Autodesk Inventor part; units mm, degrees
ref_plane "YZ Plane" through (0, 0, 0) normal (1, 0, 0) x (0, 1, 0)
ref_plane "XZ Plane" through (0, 0, 0) normal (0, 1, 0) x (-1, 0, 0)
ref_plane "XY Plane" through (0, 0, 0) normal (0, 0, 1) x (1, 0, 0)
sketch "Sketch1" plane through (0, 0, 0) normal (0, 0, 1) x (1, 0, 0)
  line L0 (0, 0) -> (2.5, 0)
  line L1 (2.5, 0) -> (2.5, 8)
  line L2 (2.5, 8) -> (0, 8)
  line L3 (0, 8) -> (0, 0)
  line L4 (2.5, 8) -> (42, 8)
  line L5 (42, 8) -> (42, 0)
  line L6 (42, 0) -> (2.5, 0)
  line L7 (2.5, 0) -> (2.5, 8)
  circle A0 centre (42, 4) radius 2.5
  point P0 (42, 1.5)
  point P1 (42, 6.5)
  dimension "d0" = 8
  dimension "d1" = 2.5
  dimension "d2" = 39.5
  dimension "d3" = 5
revolve "Revolution1" add sketch "Sketch1" angle 360 about axis through (0, 8, 0) along (0, -1, 0) contours L1 L4 L5 A0 L6
sketch "Sketch2" plane through (0, 8, 0) normal (0, 1, 0) x (1, 0, 0)
  circle A0 centre (0, 0) radius 2.5
  circle A1 centre (0, 0) radius 30
  circle A2 centre (0, 0) radius 5
  line L0 (-4.3623, -2.4434) -> (-29.9003, -2.4434)
  line L1 (-4.3623, 2.4434) -> (-29.9003, 2.4434)
  line L2 (4.3623, 2.4434) -> (29.9003, 2.4434)
  line L3 (4.3623, -2.4434) -> (29.9003, -2.4434)
  line L4 (2.0546, -4.5583) -> (2.0546, -29.9296)
  line L5 (-2.0546, -4.5583) -> (-2.0546, -29.9296)
  line L6 (-2.0546, 4.5583) -> (-2.0546, 60.5512)
  line L7 (2.0546, 4.5583) -> (2.0546, 29.9296)
  point P0 (-2.0546, 29.9296)
  dimension "d5" = 60
  dimension "d6" = 10
extrude "Extrusion1" cut sketch "Sketch2" against normal blind 25 contours L2 A2 L7 A1 | A1 L4 A2 L3 | L6 A2 L1 A1 | A1 L0 A2 L5
properties part number "Roue_pami_V3"
Work out the finished part from the listing and answer in its coordinate system (mm). A direction names the side the tool comes from. Round coordinates to 2 decimals unless told otherwise and drop trailing zeros. Loops run counter-clockwise (first coordinate to the right, second up) from the corner with the lowest first, then second, coordinate; pieces in that order, holes last.
(1) The part is cut by section A-A, the plane x = 0. Give the vertices of the cut face in (y, z), and give its area (3 significant figures).
Computed values:
outline: (0, -42) - (1.5, -42) arc R2.5 cw to (6.5, -42) - (8, -42) - (8, -2.5) - (0, -2.5) - close; (0, 2.5) - (8, 2.5) - (8, 42) - (6.5, 42) arc R2.5 cw to (1.5, 42) - (0, 42) - close
area: 612 mm2
(2) The mould has two halves that part along Z. Classify faces 3 (the cylindrical face through (40.06, 7.24, 12.62)), 4 (the cylindrical face through (-3, 4, 4)), 5 (the flat face through (9, 8, 1)): pulls with the +Z half, pulls with the -Z half, needs draft (parallel to the pull), parting line crosses it, or undercut.
Computed values:
face 3: parting line crosses it
face 4: undercut
face 5: needs draft
(3) For faces 1 (the cylindrical face through (-20.86, 4.06, -21.56)), 2 (the flat face through (9, 0, 1)), determine the directions among +Z, -Z, +X, -X, +Y, -Y from which every point of the face is accessible in a straight line to the end or side of a thin tool.
Computed values:
face 1: +Y, -Y
face 2: +Z, -Z, +X, -X, -Y
(4) Find the intervals of material crossed by L1, parallel to Z at x = 5, y = 7.5; L2, parallel to X at y = 4, z = -7; L3, parallel to Z at x = 22, y = 5.5, in increasing order.
Computed values:
L1: z = -41.7 to -29.58, -2.44 to 2.44, 29.58 to 41.7
L2: x = -38.87 to -29.17, -2.05 to 2.05, 29.17 to 38.87
L3: z = -33.41 to -20.4, -2.44 to 2.44, 20.4 to 33.41
(5) The part is cut by section C-C, the plane y = 3.75. Give the vertices of the cut face in (x, z), and give its area (3 significant figures).
Computed values:
outline: circle Ø79.03 at (0, 0); hole (-29.9, -2.44) arc R30 ccw to (-2.05, -29.93) - (-2.05, -4.56) arc R5 cw to (-4.36, -2.44) - close; hole (-29.9, 2.44) - (-4.36, 2.44) arc R5 cw to (-2.05, 4.56) - (-2.05, 29.93) arc R30 ccw to start; hole circle Ø5 at (0, 0); hole (2.05, -29.93) arc R30 ccw to (29.9, -2.44) - (4.36, -2.44) arc R5 cw to (2.05, -4.56) - close; hole (2.05, 4.56) arc R5 cw to (4.36, 2.44) - (29.9, 2.44) arc R30 ccw to (2.05, 29.93) - close
area: 2,590 mm2
(6) Each of these flat-tipped pins is pushed along its axis until it touches: P1, Ø4, axis at x = 13, y = 4, coming from the -Z side; P2, Ø4, axis at x = 0, z = 0, coming from the -Y side; P3, Ø2.5, axis at x = -22.5, y = 5, coming from the +Z side; P4, Ø4, axis at x = -32, y = 2, coming from the -Z side. Where does it stop, or does it pass through?
Computed values:
P1: stops at z = -38.44
P2: passes through
P3: stops at z = 34.28
P4: stops at z = -29.33
(7) The part is cut by section B-B, the plane z = 0. Give the vertices of the cut face in (x, y).
Computed values:
outline: (-42, 0) - (-2.5, 0) - (-2.5, 8) - (-42, 8) - (-42, 6.5) arc R2.5 cw to (-42, 1.5) - close; (2.5, 0) - (42, 0) - (42, 1.5) arc R2.5 cw to (42, 6.5) - (42, 8) - (2.5, 8) - close
(8) The part is cut by section D-D, the plane z = -13. Give the number of separate pieces and of enclosed holes in the cut face, and give its area (3 significant figures).
Computed values:
separate pieces: 3
enclosed holes: 0
area: 219 mm2
